from build123d import *

# Parameters (mm, degrees)
SKETCH2_R          = 1.25
CUT_EXTRUDE1_DEPTH = 19.25
FILLET1_R          = 2
SKETCH3_R          = 2.5
CUT_EXTRUDE2_DEPTH = 13.25
SKETCH4_R          = 4.65
CUT_EXTRUDE3_DEPTH = 10


with BuildPart() as part:
    # Sketch1 → Revolve1 (revolve)
    with BuildSketch(Plane(origin=(0, 0, 0), x_dir=(1, 0, 0), z_dir=(0, 1, 0))):
        Polygon((-6.130434783, 14.45), (6.626387667, 14.45), (10.619565217, 11.440924884), (10.619565217, 4), (14.619565217, 4), (14.619565217, 0), (13.372742768, 0), (-6.130434783, 0), (-7.630434783, 0), (-7.630434783, 18.25), (-6.130434783, 18.25), align=None)
    revolve(axis=Axis((-12.391304348, 0, 0), (1, 0, 0)))

    # Sketch2 → Cut-Extrude1 (cut, through all)
    with BuildSketch(Plane(origin=(10.619565217, 0, 0), x_dir=(0, 0, -1), z_dir=(1, 0, 0))):
        with Locations((0, 9.5)):
            Circle(SKETCH2_R)
        with Locations((6.717514421, 6.717514421)):
            Circle(SKETCH2_R)
        with Locations((9.5, 0)):
            Circle(SKETCH2_R)
        with Locations((6.717514421, -6.717514421)):
            Circle(SKETCH2_R)
        with Locations((0, -9.5)):
            Circle(SKETCH2_R)
        with Locations((-6.717514421, -6.717514421)):
            Circle(SKETCH2_R)
        with Locations((-9.5, 0)):
            Circle(SKETCH2_R)
        with Locations((-6.717514421, 6.717514421)):
            Circle(SKETCH2_R)
    extrude(amount=-CUT_EXTRUDE1_DEPTH, mode=Mode.SUBTRACT)

    # Fillet1
    fillet1_edges = [part.edges().sort_by_distance(p)[0] for p in [
        (14.619565217, 0, 4),
    ]]
    fillet(fillet1_edges, radius=FILLET1_R)

    # Sketch3 → Cut-Extrude2 (cut)
    with BuildSketch(Plane.ZY.offset(7.630434783)):
        with Locations((0, 9.5)):
            Circle(SKETCH3_R)
        with Locations((6.717514421, 6.717514421)):
            Circle(SKETCH3_R)
        with Locations((9.5, 0)):
            Circle(SKETCH3_R)
        with Locations((6.717514421, -6.717514421)):
            Circle(SKETCH3_R)
        with Locations((0, -9.5)):
            Circle(SKETCH3_R)
        with Locations((-6.717514421, -6.717514421)):
            Circle(SKETCH3_R)
        with Locations((-9.5, 0)):
            Circle(SKETCH3_R)
        with Locations((-6.717514421, 6.717514421)):
            Circle(SKETCH3_R)
    extrude(amount=-CUT_EXTRUDE2_DEPTH, mode=Mode.SUBTRACT)

    # Sketch4 → Cut-Extrude3 (cut)
    with BuildSketch(Plane.ZY.offset(7.630434783)):
        Circle(SKETCH4_R)
    extrude(amount=-CUT_EXTRUDE3_DEPTH, mode=Mode.SUBTRACT)


solid = part.part
Geometry check sheet. Reference: the model listing, model coordinates, mm. A direction names the side the tool comes from. Give positions to 0.01 mm unless a question says otherwise; leave off trailing zeros.
1) Tool access check on faces 5 (the cylindrical face through (8.155, -8.446, -0.672)), 6 (the flat face through (5.62, -1, -11)), 7 (the flat face through (10.62, -5, 0)). Record the directions out of +Z, -Z, +X, -X, +Y, -Y that give a thin tool (end or side, any length) a straight path to the whole face; none if there is none.
Results are:
face 5: +X, -X
face 6: -X
face 7: +X
2) Cross-section at A-A (x = -4). Give the number of separate pieces and of enclosed holes in the cut face, then the cut area to 3 significant figures.
Results are:
separate pieces: 1
enclosed holes: 9
area: 431 mm2
3) Gauge pin test, flat ends, axial feed: pin 1 (4 mm diameter, centred on x = 11.5, z = 5, fed in from -Y); pin 2 (6 mm diameter, centred on x = -1, z = 7, fed in from +Y); pin 3 (8 mm diameter, centred on x = -0.5, y = 8.5, fed in from -Z). Record the tip position at first contact, or that the pin passes through.
Results are:
pin 1: stops at y = -11.41
pin 2: stops at y = 13.89
pin 3: stops at z = -13.73
4) Draft check along Y on faces 1 (the flat face through (-6.13, 10, 11)), 2 (the flat face through (5.62, -8, 8)), 3 (the conical face through (10.43, -11.31, 2.51)), 4 (the cylindrical face through (-1, 0, 7)). Enter one of: released by +Y, released by -Y, zero draft, split by the parting line, or undercut.
Results are:
face 1: zero draft
face 2: undercut
face 3: split by the parting line
face 4: undercut
5) Material ranges on probe 1 along Y at (x, z) = (-2.5, -1); probe 2 along Y at (x, z) = (8.75, 0); probe 3 along Z at (x, y) = (4, -8.5), recorded low to high.
Results are:
probe 1: y = -14.42 to -11.79, -7.21 to -4.54, 4.54 to 7.21, 11.79 to 14.42
probe 2: y = -12.85 to -10.75, -8.25 to 8.25, 10.75 to 12.85
probe 3: z = -11.69 to -8.47, -4.96 to -2.29, 2.29 to 4.96, 8.47 to 11.69
